Part model, mm, in its own coordinate system. Coordinates: 2 decimals unless noted, no trailing zeros. Write each loop counter-clockwise with the first axis right and the second up, starting at its lowest first coordinate (ties: lowest second). Pieces come first, ordered by that corner, then holes. Notation, with made-up numbers: M -34,-31 L 24,-31 A17 cw 24,-21 Z; hole C -14.5,-12 d10. An arc over 180 degrees is marked long. Use a Markdown table: item, result. Add a question column.
Q1. Wall check: L1, parallel to X at y = -1.5, z = -239.5 (3 decimals); L2, parallel to X at y = -4.5, z = -43.5 (3 decimals); L3, parallel to Z at x = -57.5, y = -2 (3 decimals). Give the ranges that are in metal, low to high. Write a range as from..to.
Q2. Slice it at B-B on x = -199. Write the cut outline in (y, z), then the cut area to 3 significant figures.
Q3. Slice it at A-A on z = 261. Write the cut outline in (x, y).
Q4. Pin check, flat tip, straight feed: pin 1 Ø2 at (y, z) = (-4, 186) entering from +X (3 decimals). Stop position of the tip, or through.
Q5. Slice it at C-C on y = -5.25. Write the cut outline in (x, z).
from build123d import *

# Parameters (mm, degrees)
F0_W     = 609.6
F0_H     = 609.6
F1_DEPTH = 6.35
F2_SIZE2 = 5.08
F2_SIZE  = 12.7


with BuildPart() as f1:
    # F0 (on Front) → F1 (new body)
    with BuildSketch(Plane.XZ):
        Rectangle(F0_W, F0_H)
    extrude(amount=F1_DEPTH)

    # F2
    f2_edges = [f1.edges().sort_by_distance(p)[0] for p in [
        (304.8, -6.35, 0),
        (0, -6.35, 304.8),
        (-304.8, -6.35, 0),
        (0, -6.35, -304.8),
    ]]
    f2_side = f1.faces().sort_by_distance((0, -6.35, 0))[0]
    chamfer(f2_edges, length=F2_SIZE, length2=F2_SIZE2, reference=f2_side)


solid = f1.part
Recorded:
| question | item | result |
|---|---|---|
| 1 | L1 | -304.225..304.225 |
| 1 | L2 | -296.725..296.725 |
| 1 | L3 | -302.975..302.975 |
| 2 | outline | M -6.35,-292.1 L -1.27,-304.8 L 0,-304.8 L 0,304.8 L -1.27,304.8 L -6.35,292.1 Z |
| 2 | area | 3,810 mm² |
| 3 | outline | M -304.8,-1.27 L -292.1,-6.35 L 292.1,-6.35 L 304.8,-1.27 L 304.8,0 L -304.8,0 Z |
| 4 | pin 1 | x = 300.475 |
| 5 | outline | M -294.85,-294.85 L 294.85,-294.85 L 294.85,294.85 L -294.85,294.85 Z |
